Source: CAD feature listing. Evaluate the final solid. Frame: model axes, mm. Coordinates: 2 decimals unless noted, no trailing zeros. Write each loop counter-clockwise with the first axis right and the second up, starting at its lowest first coordinate (ties: lowest second). Pieces come first, ordered by that corner, then holes. Notation, with made-up numbers: M -16.5,2 L 22.5,2 A21 cw 22.5,41 Z; hole C 1,86.5 d1. An arc over 180 degrees is marked long. Write item = value, one per line. Start each with the question number.
1. Pull-direction query (Y, two-part tool) for faces 1 (the face through (-9.64, 29.26, 0.99)), 2 (the face through (-8, 37.391, 1)), 3 (the face through (-7, 7.541, 1)), 4 (the face through (-7, 19, 0)); classes: pulls with the +Y half, pulls with the -Y half, needs draft (parallel to the pull), parting line crosses it, or undercut.
2. Section query B-B (x = -10.5). Output: boundary loops of the cut face in (y, z), then the cut area to 3 significant figures.
3. Section query A-A (y = 25.5). Output: boundary loops of the cut face in (x, z).
4. Line query: line 1 along X through (y, z) = (20.5, 0.4); line 2 along Y through (x, z) = (-11, 1.55); line 3 along Y through (x, z) = (-10.5, 1.9). Output: solid intervals per line, ascending.
5. Section query C-C (z = 1.25). Output: boundary loops of the cut face in (x, y).
```python
from build123d import *

# Parameters (mm, degrees)
SKETCH1_R           = 5.034687392
BOSS_EXTRUDE1_DEPTH = 2


with BuildPart() as part:
    # Sketch1 → Boss-Extrude1 (new body)
    with BuildSketch(Plane.XY):
        Polygon((29.741294814, 7.540555765), (-45.258705186, 7.540555765), (-45.258705186, 37.390988743), (29.741294814, 37.390955861), align=None)
        with Locations((-8.98326267, 24.266867238)):
            Circle(SKETCH1_R, mode=Mode.SUBTRACT)
    extrude(amount=BOSS_EXTRUDE1_DEPTH)


solid = part.part
```
Results are:
q1.face_1 = undercut
q1.face_2 = pulls with the +Y half
q1.face_3 = pulls with the -Y half
q1.face_4 = needs draft
q2.outline = M 7.54,0 L 19.47,0 L 19.47,2 L 7.54,2 Z; M 29.07,0 L 37.39,0 L 37.39,2 L 29.07,2 Z
q2.area = 40.5 mm^2
q3.outline = M -45.26,0 L -13.86,0 L -13.86,2 L -45.26,2 Z; M -4.1,0 L 29.74,0 L 29.74,2 L -4.1,2 Z
q4.line_1 = -45.26 to -12.32, -5.64 to 29.74
q4.line_2 = 7.54 to 19.65, 28.88 to 37.39
q4.line_3 = 7.54 to 19.47, 29.07 to 37.39
q5.outline = M -45.26,7.54 L 29.74,7.54 L 29.74,37.39 L -45.26,37.39 Z; hole C -8.98,24.27 d10.07
